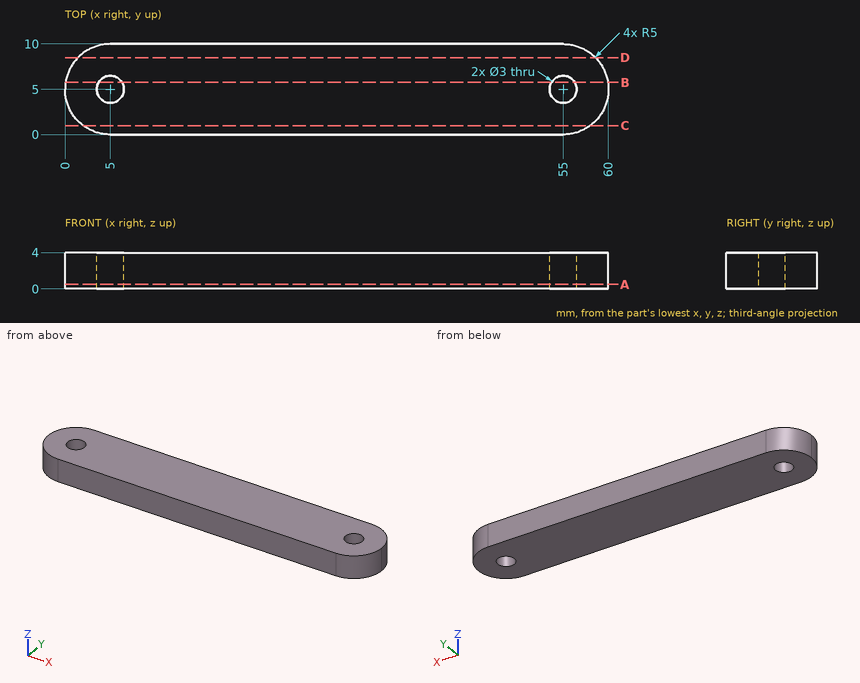
Geometry check sheet. Reference: drawing and pictorial views, mm from the part's lowest x, y, z. Coordinates: 2 decimals unless noted, no trailing zeros. Write each loop counter-clockwise with the first axis right and the second up, starting at its lowest first coordinate (ties: lowest second). Pieces come first, ordered by that corner, then holes. Notation, with made-up numbers: M -17.5,25.25 L 10.5,25.25 A33 cw 10.5,62.25 Z; hole C 28,-23 d8. An arc over 180 degrees is marked long. Write item = value, one per line. Start each with the question number.
1. Sectioned sample at D-D (y = 8.5). Record the cut outline in (x, z).
2. Sectioned sample at A-A (z = 0.5). State how many separate pieces and enclosed holes the cut face has.
3. Sectioned sample at C-C (y = 1). Record the cut outline in (x, z), then the cut area to 3 significant figures.
4. Thickness scan on probe 1 along X at (y, z) = (5, 2.9); probe 2 along Y at (x, z) = (5, 1.05); probe 3 along X at (y, z) = (4.5, 3.35) (1 decimal). Record the ranges inside material, lowest first.
5. Go/stop test with a flat-tipped pin: pin 1 (1.5 mm diameter, centred on y = 6, z = 1.5, fed in from -X). Record where the tip stops, or that it passes through.
6. Sectioned sample at B-B (y = 5.75). Record the cut outline in (x, z).
The answers:
q1.outline = M 1.43,0 L 58.57,0 L 58.57,4 L 1.43,4 Z
q2.separate_pieces = 1
q2.enclosed_holes = 2
q3.outline = M 2,0 L 58,0 L 58,4 L 2,4 Z
q3.area = 224 mm²
q4.probe_1 = 0 to 3.5, 6.5 to 53.5, 56.5 to 60
q4.probe_2 = 0 to 3.5, 6.5 to 10
q4.probe_3 = 0 to 3.6, 6.4 to 53.6, 56.4 to 60
q5.pin_1 = 0.01
q6.outline = M 0.06,0 L 3.7,0 L 3.7,4 L 0.06,4 Z; M 6.3,0 L 53.7,0 L 53.7,4 L 6.3,4 Z; M 56.3,0 L 59.94,0 L 59.94,4 L 56.3,4 Z
